For this review, take the finished solid that the model builds, in its own axes (mm). A direction names the side the tool comes from. Round coordinates to 2 decimals unless told otherwise and drop trailing zeros. Loops run counter-clockwise (first coordinate to the right, second up) from the corner with the lowest first, then second, coordinate; pieces in that order, holes last.
1) Insertion check: pin 1 (2 mm diameter, centred on x = 1.5, y = -2, fed in from +Z); pin 2 (0.8 mm diameter, centred on y = 0, z = 1, fed in from +X). Each pin has a flat end and moves straight along its axis. Give the tip position at first contact, or say it passes through.
2) Take a section at B-B (x = 0). State the section outline as (y, z) points, then the cut area to 3 significant figures.
3) Tool access review of faces 1 (the cylindrical face through (-0.05, -2.45, 1.17)), 2 (the flat face through (0, 0, 1.6)), 3 (the cylindrical face through (0.05, 2.45, 1.17)): name each direction out of +Z, -Z, +X, -X, +Y, -Y from which nothing blocks a thin tool from reaching the whole face with its end or side.
4) Wall thickness on L1, parallel to X at y = -0.1, z = 1.35; L2, parallel to X at y = 0.9, z = 1.3; L3, parallel to Y at x = 0.8, z = 0.45: over which ranges is each line inside the solid? List them lowest first.
5) Take a section at D-D (z = 0.5). State the section outline as (x, y) points, then the cut area to 3 significant figures.
6) Take a section at A-A (z = 1.4). State the section outline as (x, y) points (3 decimals).
```python
from build123d import *

# Parameters (mm, degrees)
SKETCH_R     = 2.45
PAD_DEPTH    = 1.6
SKETCH001_W  = 4.9
SKETCH001_H  = 0.75
PAD001_DEPTH = 1.6
SKETCH002_R  = 3
PAD002_DEPTH = 0.75
FILLET_R     = 0.5


with BuildPart() as part:
    # Sketch → Pad (new body)
    with BuildSketch(Plane.XY):
        Circle(SKETCH_R)
    extrude(amount=PAD_DEPTH)

    # Sketch001 → Pad001 (join)
    with BuildSketch(Plane.XY):
        Rectangle(SKETCH001_W, SKETCH001_H)
    extrude(amount=PAD001_DEPTH)

    # Sketch002 → Pad002 (join)
    with BuildSketch(Plane.XY):
        Circle(SKETCH002_R)
    extrude(amount=PAD002_DEPTH)

    # Fillet
    fillet_edges = [part.edges().sort_by_distance(p)[0] for p in [
        (-3, 0, 0.75),
    ]]
    fillet(fillet_edges, radius=FILLET_R)


solid = part.part
```
Response:
1. pin 1: stops at z = 1.6
1. pin 2: stops at x = 2.86
2. outline: (-3, 0) - (3, 0) - (3, 0.25) arc R0.5 ccw to (2.5, 0.75) - (2.45, 0.75) - (2.45, 1.6) - (-2.45, 1.6) - (-2.45, 0.75) - (-2.5, 0.75) arc R0.5 ccw to (-3, 0.25) - close
2. area: 8.56 mm2
3. face 1: +Z, -Y
3. face 2: +Z, +X, -X, +Y, -Y
3. face 3: +Z, +Y
4. L1: x = -2.45 to 2.45
4. L2: x = -2.28 to 2.28
4. L3: y = -2.85 to 2.85
5. outline: circle Ø5.87 at (0, 0)
5. area: 27.0 mm2
6. outline: (-2.45, -0.375) - (-2.421, -0.375) arc R2.45 ccw to (2.421, -0.375) - (2.45, -0.375) - (2.45, 0.375) - (2.421, 0.375) arc R2.45 ccw to (-2.421, 0.375) - (-2.45, 0.375) - close
